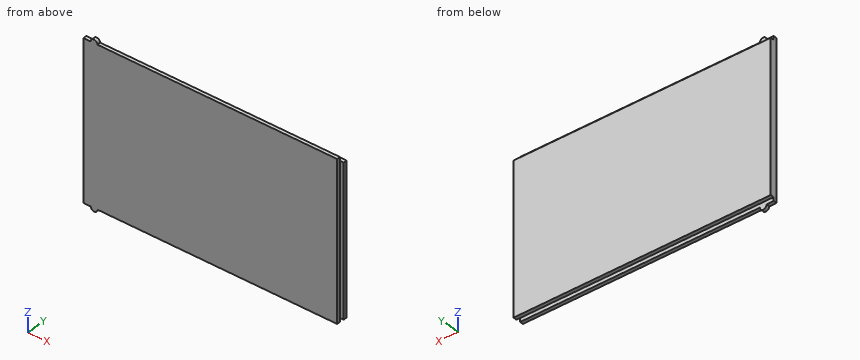
Autodesk Inventor part; units mm, degrees
ref_plane "YZ Plane" through (0, 0, 0) normal (1, 0, 0) x (0, 1, 0)
ref_plane "XZ Plane" through (0, 0, 0) normal (0, 1, 0) x (-1, 0, 0)
ref_plane "XY Plane" through (0, 0, 0) normal (0, 0, 1) x (1, 0, 0)
sketch "Sketch1" plane through (0, 0, 0) normal (0, 1, 0) x (-1, 0, 0)
  line L0 (-36.727, -18.0642) -> (-36.727, 22.633)
  line L1 (-36.727, 22.633) -> (28.3668, 22.633)
  line L2 (28.3668, -18.0642) -> (-36.727, -18.0642)
  line L3 (30.2718, 23.5855) -> (28.3559, 23.5855)
  arc A0 (28.3559, 23.5855) -> (26.5779, 23.5855) centre (27.4669, 23.5855) ccw
  line L4 (26.5779, 23.5855) -> (-37.6795, 23.5855)
  line L5 (-37.6795, 23.5855) -> (-37.6795, -19.0167)
  line L6 (-37.6795, -19.0167) -> (26.5779, -19.0167)
  arc A1 (26.5779, -19.0167) -> (28.3559, -19.0167) centre (27.4669, -19.0167) ccw
  line L7 (28.3559, -19.0167) -> (30.2718, -19.0167)
  line L8 (30.2718, -18.6357) -> (27.8029, -18.6357)
  line L9 (27.1309, -18.6357) -> (-37.2985, -18.6357)
  line L10 (-37.2985, -18.6357) -> (-37.2985, 23.2045)
  line L11 (-37.2985, 23.2045) -> (27.1309, 23.2045)
  line L12 (27.8029, 23.2045) -> (30.2718, 23.2045)
  arc A2 (26.5779, -18.6357) -> (28.3559, -18.6357) centre (27.4669, -18.6524) ccw
  arc A3 (28.3559, 23.2045) -> (26.5779, 23.2045) centre (27.4669, 23.2045) ccw
  line L13 (30.2718, -18.6357) -> (30.2718, 23.2045)
  point P0 (0, 0)
  point P1 (25.8871, -17.6673)
  dimension "d0" = 0.381
  dimension "d1" = 0.889
extrude "Extrusion1" add sketch "Sketch1" along normal blind 0.9144
sketch "Sketch2" plane through (0, 0.9144, 0) normal (0, 1, 0) x (1, 0, 0)
  line L0 (37.2985, 18.6357) -> (-26.5779, 18.6357)
  line L1 (-26.5779, -23.2045) -> (37.2985, -23.2045)
  line L2 (37.2985, 17.6451) -> (-26.5779, 17.6451)
  line L3 (-26.5779, -22.2139) -> (37.2985, -22.2139)
  line L4 (-26.5779, 17.6451) -> (-30.2718, 17.6451)
  line L5 (-30.2718, 18.6357) -> (-30.2718, -23.2045)
  line L6 (-26.5779, -22.2139) -> (-30.2718, -22.2139)
  line L7 (37.2985, 17.6451) -> (38.251, 17.6451)
  line L8 (38.251, 17.6451) -> (38.251, -22.2139)
  line L9 (38.251, -22.2139) -> (37.2985, -22.2139)
  point P0 (0, 0)
  dimension "d4" = 0.9906
  dimension "d5" = 0.9906
  dimension "d6" = 0.9525
extrude "Extrusion2" add sketch "Sketch2" along normal blind 0.9652
properties part number "ControllerLid"
Could you check a few things on this model? Use its own coordinates, in mm. Coordinates: 2 decimals unless noted, no trailing zeros. Loops run counter-clockwise (first coordinate to the right, second up) from the corner with the lowest first, then second, coordinate; pieces in that order, holes last.
1. For P1, Ø0.9, axis at x = 18.5, z = 23, coming from the +Y side; P2, Ø1, axis at x = -29, y = 0.5, coming from the +Z side; P3, Ø0.5, axis at x = 5.5, y = 0.5, coming from the -Z side, each with a flat end and sliding along its axis, tell me the tip position at first contact or that it passes through.
2. Imagine slicing it at B-B (y = 1.45). Please give me the cut outline in (x, z), and give its area (3 significant figures).
3. I need wall thicknesses on L1, parallel to Z at x = -1, y = 1.45; L2, parallel to Z at x = 22, y = 0.75; L3, parallel to X at y = 0.35, z = 19. Which ranges of each line are inside material? Lowest first, please.
4. Imagine slicing it at A-A (x = -12.5). Please give me the cut outline in (y, z), and give its area (3 significant figures).
Computed values:
1. P1: stops at y = 0.91
1. P2: stops at z = 23.2
1. P3: stops at z = -18.64
2. outline: (-30.27, -17.65) - (38.25, -17.65) - (38.25, 22.21) - (-30.27, 22.21) - close
2. area: 2,730 mm2
3. L1: z = -17.65 to 22.21
3. L2: z = -18.64 to 23.2
3. L3: x = -30.27 to 37.3
4. outline: (0, -18.64) - (0.91, -18.64) - (0.91, -17.65) - (1.88, -17.65) - (1.88, 22.21) - (0.91, 22.21) - (0.91, 23.2) - (0, 23.2) - close
4. area: 76.7 mm2
